Geometry check sheet. Reference: the model listing, model coordinates, mm. A direction names the side the tool comes from. Give positions to 0.01 mm unless a question says otherwise; leave off trailing zeros. Order: outer loops, then holes, each group sorted by start corner. A loop starts at its lowest first (then second) coordinate and runs counter-clockwise, first axis right, second up.
from build123d import *

# Parameters (mm, degrees)
SKETCH1_R           = 0.95
BOSS_EXTRUDE1_DEPTH = 4
SKETCH2_W           = 16.2
SKETCH2_H           = 14.645
CUT_EXTRUDE1_DEPTH  = 2


with BuildPart() as part:
    # Sketch1 → Boss-Extrude1 (new body)
    with BuildSketch(Plane.XY):
        with BuildLine():
            Line((2, 14.645), (14.2, 14.645))
            ThreePointArc((14.2, 14.645), (15.614213562, 14.059213562), (16.2, 12.645))
            Line((16.2, 12.645), (16.2, 8.3225))
            Line((16.2, 8.3225), (12.2, 8.3225))
            Line((12.2, 8.3225), (12.2, 6.3225))
            Line((12.2, 6.3225), (16.2, 6.3225))
            Line((16.2, 6.3225), (16.2, 2))
            ThreePointArc((16.2, 2), (15.614213562, 0.585786438), (14.2, 0))
            Line((14.2, 0), (2, 0))
            ThreePointArc((2, 0), (0.585786438, 0.585786438), (0, 2))
            Line((0, 2), (0, 6.3225))
            Line((0, 6.3225), (4, 6.3225))
            Line((4, 6.3225), (4, 8.3225))
            Line((4, 8.3225), (0, 8.3225))
            Line((0, 8.3225), (0, 12.645))
            ThreePointArc((0, 12.645), (0.585786438, 14.059213562), (2, 14.645))
        make_face()
        with Locations((2.75, 12.145)):
            Circle(SKETCH1_R, mode=Mode.SUBTRACT)
        with Locations((13.45, 2.5)):
            Circle(SKETCH1_R, mode=Mode.SUBTRACT)
        with Locations((13.45, 12.145)):
            Circle(SKETCH1_R, mode=Mode.SUBTRACT)
        with Locations((2.75, 2.5)):
            Circle(SKETCH1_R, mode=Mode.SUBTRACT)
    extrude(amount=BOSS_EXTRUDE1_DEPTH)

    # Sketch2 → Cut-Extrude1 (cut)
    with BuildSketch(Plane(origin=(0, 0, 0), x_dir=(-1, 0, 0), z_dir=(0, 0, -1))):
        with Locations((-8.1, 7.3225)):
            Rectangle(SKETCH2_W, SKETCH2_H)
    extrude(amount=-CUT_EXTRUDE1_DEPTH, mode=Mode.SUBTRACT)


solid = part.part
Item 1: Set-up check for faces 5 (the flat face through (12.2, 7, 3)), 6 (the flat face through (2, 6.322, 3)), 7 (the flat face through (8, 14.645, 3)): record each of +Z, -Z, +X, -X, +Y, -Y from which the full face is reachable in a straight line by a thin tool's end or side.
Reported:
face 5: +Z, -Z, +X
face 6: +Z, -Z, -X
face 7: +Z, -Z, +X, -X, +Y
Item 2: Scan lines: L1, parallel to X at y = 2.5, z = 3.35; L2, parallel to Y at x = 14, z = 3.95 (1 decimal); L3, parallel to Y at x = 12.25, z = 2.1 (1 decimal). Record each from-to range of solid material in increasing order.
Reported:
L1: x = 0 to 1.8, 3.7 to 12.5, 14.4 to 16.2
L2: y = 0 to 1.7, 3.3 to 6.3, 8.3 to 11.4, 12.9 to 14.6
L3: y = 0 to 6.3, 8.3 to 14.6
Item 3: Gauge pin test, flat ends, axial feed: pin 1 (0.6 mm diameter, centred on y = 7.5, z = 3, fed in from +X); pin 2 (0.6 mm diameter, centred on y = 7, z = 3, fed in from -X). Record the tip position at first contact, or that the pin passes through.
Reported:
pin 1: stops at x = 12.2
pin 2: stops at x = 4
Item 4: Sectioned sample at D-D (x = 1.25). Enter the section's corners in (y, z), and give its area (3 significant figures).
Reported:
outline: (0.15, 2) - (6.32, 2) - (6.32, 4) - (0.15, 4) - close; (8.32, 2) - (14.5, 2) - (14.5, 4) - (8.32, 4) - close
area: 24.7 mm2
Item 5: Sectioned sample at B-B (y = 2.5). Enter the section's corners in (x, z).
Reported:
outline: (0, 2) - (1.8, 2) - (1.8, 4) - (0, 4) - close; (3.7, 2) - (12.5, 2) - (12.5, 4) - (3.7, 4) - close; (14.4, 2) - (16.2, 2) - (16.2, 4) - (14.4, 4) - close
Item 6: Draft check along Y on faces 1 (the cylindrical face through (0.6, 0.57, 2.99)), 2 (the flat face through (0, 4, 3)), 3 (the cylindrical face through (14.356, 12.43, 2.986)), 4 (the cylindrical face through (2.05, 12.79, 2.99)). Enter one of: released by +Y, released by -Y, zero draft, split by the parting line, or undercut.
Reported:
face 1: released by -Y
face 2: zero draft
face 3: undercut
face 4: undercut
Item 7: Sectioned sample at A-A (x = 13.45). Give the number of separate pieces and of enclosed holes in the cut face, and give its area (3 significant figures).
Reported:
separate pieces: 4
enclosed holes: 0
area: 17.7 mm2
